Autodesk Inventor part; units mm, degrees
ref_plane "YZ Plane" through (0, 0, 0) normal (1, 0, 0) x (0, 1, 0)
ref_plane "XZ Plane" through (0, 0, 0) normal (0, 1, 0) x (-1, 0, 0)
ref_plane "XY Plane" through (0, 0, 0) normal (0, 0, 1) x (1, 0, 0)
sketch "Sketch2" plane through (0, 0, 0) normal (0, 1, 0) x (-1, 0, 0)
  line L0 (-89, 99) -> (89, 99)
  line L1 (89, 99) -> (89, -99)
  line L2 (89, -99) -> (-89, -99)
  line L3 (-89, -99) -> (-89, 99)
  line L4 (-89, 99) -> (89, -99) construction
  line L5 (89, 99) -> (-89, -99) construction
  line L6 (-89, 99) -> (89, 99)
  line L7 (89, 99) -> (89, -81)
  line L8 (89, -81) -> (-89, -81)
  line L9 (-89, -81) -> (-89, 99)
  line L10 (-4.5, 99) -> (-89, 99)
  line L11 (-89, 99) -> (-89, 46)
  line L12 (-89, 46) -> (-4.5, 46)
  line L13 (-4.5, 46) -> (-4.5, 99)
  line L14 (4.5, 99) -> (89, 99)
  line L15 (89, 99) -> (89, 46)
  line L16 (89, 46) -> (4.5, 46)
  line L17 (4.5, 46) -> (4.5, 99)
  line L18 (22.5, 77.5) -> (22.5, 66.5)
  line L19 (16.5, 66.5) -> (16.5, 77.5)
  line L20 (-22.5, 66.5) -> (-22.5, 77.5)
  line L21 (-16.5, 77.5) -> (-16.5, 66.5)
  line L22 (-22.5, 99) -> (-16.5, 99)
  line L23 (-16.5, 99) -> (-16.5, 46)
  line L24 (-16.5, 46) -> (-22.5, 46)
  line L25 (-22.5, 46) -> (-22.5, 99)
  line L26 (16.5, 99) -> (22.5, 99)
  line L27 (22.5, 99) -> (22.5, 46)
  line L28 (22.5, 46) -> (16.5, 46)
  line L29 (16.5, 46) -> (16.5, 99)
  line L30 (-89, 99) -> (89, 99)
  line L31 (89, 99) -> (89, 98)
  line L32 (89, 98) -> (-89, 98)
  line L33 (-89, 98) -> (-89, 99)
  line L34 (89, -81) -> (74, -81)
  line L35 (74, -81) -> (74, -65)
  line L36 (74, -65) -> (89, -65)
  line L37 (89, -65) -> (89, -81)
  line L38 (-89, -81) -> (-74, -81)
  line L39 (-74, -81) -> (-74, -65)
  line L40 (-74, -65) -> (-89, -65)
  line L41 (-89, -65) -> (-89, -81)
  point P0 (0, 0)
  point P1 (4.5, 99)
  point P2 (-4.5, 99)
  point P3 (-89, 46)
  point P4 (89, 46)
  point P5 (4.5, 98)
  point P6 (-4.5, 98)
  point P7 (-16.5, 98)
  point P8 (-22.5, 98)
  point P9 (22.5, 98)
  point P10 (16.5, 98)
  dimension "d8" = 178
  dimension "d9" = 198
  dimension "d10" = 18
  dimension "d11" = 84.5
  dimension "d12" = 53
  dimension "d13" = 84.5
  dimension "d14" = 53
  dimension "d17" = 9
  dimension "d18" = 1
  dimension "d19" = 15
  dimension "d20" = 16
  dimension "d21" = 15
  dimension "d22" = 16
extrude "Extrusion2" add sketch "Sketch2" along normal blind 3 contours L32 L23 L21 L12 L25 L20 | L12 L13 L32 L17 L16 L1 L36 L35 L8 L39 L40 L3 | L32 L27 L18 L16 L29 L19
fillet "Fillet1" radius 3 6 edges at (22.5, 1.5, 46) (-22.5, 1.5, 46) (-16.5, 1.5, 46) (-4.5, 1.5, 46) (4.5, 1.5, 46) (16.5, 1.5, 46)
fillet "Fillet2" radius 3 2 edges at (74, 1.5, -65) (-74, 1.5, -65)
sketch "Sketch5" plane through (0, 0, 0) normal (0, -1, 0) x (1, 0, 0)
  circle A0 centre (64.5, -73) radius 1.2295
  circle A1 centre (21.5, -73) radius 1.2295
  circle A2 centre (-21.5, -73) radius 1.2295
  circle A3 centre (-64.5, -73) radius 1.2295
  point P0 (0, 0)
hole "Hole2" at (64.5, 0, -73) at (21.5, 0, -73) at (-21.5, 0, -73) at (-64.5, 0, -73) direction (0, 1, 0) diameter 3.6 end through all countersink diameter 6.5 countersink angle 90
equation "\"d11\" = d13"
properties part number "base" material "Aluminum 6061"
Verification items for the finished model (mm, model axes). Coordinates: 2 decimals unless noted, no trailing zeros. Order: outer loops, then holes, each group sorted by start corner. A loop starts at its lowest first (then second) coordinate and runs counter-clockwise, first axis right, second up.
1. Sectioned sample at B-B, the plane y = 0.6. Give the number of separate pieces and of enclosed holes in the cut face, and give its area (3 significant figures).
Results found:
separate pieces: 1
enclosed holes: 4
area: 23,100 mm2
2. Sectioned sample at A-A, the plane z = 54. Record the cut outline in (x, y), and give its area (3 significant figures).
Results found:
outline: (-22.5, 0) - (-16.5, 0) - (-16.5, 3) - (-22.5, 3) - close; (-4.5, 0) - (4.5, 0) - (4.5, 3) - (-4.5, 3) - close; (16.5, 0) - (22.5, 0) - (22.5, 3) - (16.5, 3) - close
area: 63.0 mm2
3. Scan lines: line 1 (X direction, y = 2, z = -73); line 2 (X direction, y = 2.45, z = 90.5); line 3 (Z direction, x = -64.5, y = 2.2). Record each from-to range of solid material in increasing order.
Results found:
line 1: x = -74 to -66.3, -62.7 to -23.3, -19.7 to 19.7, 23.3 to 62.7, 66.3 to 74
line 2: x = -22.5 to -16.5, -4.5 to 4.5, 16.5 to 22.5
line 3: z = -81 to -74.8, -71.2 to 46
4. Go/stop test with flat-tipped pins: pin 1 Ø0.9 at (x, y) = (-54.5, 1.5) entering from +Z; pin 2 Ø0.9 at (y, z) = (2, 65.5) entering from -X; pin 3 Ø2 at (x, z) = (-21.5, -73) entering from +Y; pin 4 Ø4.5 at (x, z) = (-64.5, -73) entering from -Y. Record where each tip stops, or that it passes through.
Results found:
pin 1: stops at z = 46
pin 2: stops at x = -22.5
pin 3: passes through
pin 4: stops at y = 1
5. Sectioned sample at C-C, the plane x = 49. Record the cut outline in (y, z), and give its area (3 significant figures).
Results found:
outline: (0, -81) - (3, -81) - (3, 46) - (0, 46) - close
area: 381 mm2
